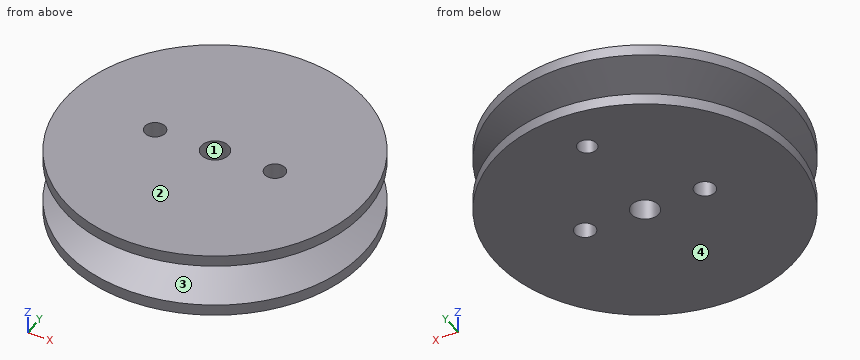
Autodesk Inventor part; units mm, degrees
ref_plane "Belt Plane" through (0, 32.131, 9.525) normal (0, 0, 1) x (1, 0, 0)
ref_plane "YZ Plane" through (0, 0, 0) normal (1, 0, 0) x (0, 1, 0)
ref_plane "XZ Plane" through (0, 0, 0) normal (0, 1, 0) x (-1, 0, 0)
sketch "Main Sketch" plane through (0, 0, 0) normal (1, 0, 0) x (0, 1, 0)
  line L0 (0, 19.05) -> (43.815, 19.05)
  line L1 (43.815, 19.05) -> (43.815, 15.8043)
  line L2 (43.815, 15.8043) -> (32.131, 12.2321)
  line L3 (32.131, 12.2321) -> (32.131, 6.8179)
  line L4 (32.131, 6.8179) -> (43.815, 3.2457)
  line L5 (43.815, 3.2457) -> (43.815, 0)
  line L6 (43.815, 0) -> (0, 0)
  line L7 (40.64, 14.8336) -> (40.64, 4.2164) construction
  line L8 (32.131, 9.525) -> (40.64, 9.525) construction
  line L9 (43.815, 15.8043) -> (43.815, 3.2457)
  line L10 (0, -4) -> (0, 24)
  line L11 (0, 0) -> (0, 19.05)
  dimension "d0" = 10.6172
  dimension "d1" = 34
  dimension "d2" = 3.175
  dimension "d6" = 19.05
  dimension "d21" = 81.28
  dimension "d25" = 11.684
  dimension "d27" = 9.525
ref_plane "Belt Plane" through (0, 32.131, 9.525) normal (0, 0, 1) x (1, 0, 0)
revolve "Body" add sketch "Main Sketch" angle 360 about axis through (0, 0, -10) along (0, 0, 1)
revolve "Groove" cut sketch "Main Sketch" angle 360 about axis through (0, 0, -10) along (0, 0, 1) contours L9 L4 L3 L2
fillet "Fillet External" [suppressed]
fillet "Fillet Internal" [suppressed]
pattern_of_one "Groove Pattern"
sketch "Sketch2" plane through (0, 0, 0) normal (0, 0, -1) x (-1, 0, 0)
  circle A0 centre (0, 0) radius 43.815
  line L0 (0, 0) -> (0, 30) construction
  circle A1 centre (0, 30) radius 2.75
  dimension "d28" = 5.5
  dimension "d29" = 30
extrude "Extrusion1" cut sketch "Sketch2" against normal blind 5 contours A1
sketch "Sketch3" plane through (0, 0, 19.05) normal (0, 0, 1) x (1, 0, 0)
  circle A0 centre (0, 0) radius 43.815
  circle A1 centre (0, 0) radius 4
  line L0 (-17.5, 0) -> (17.5, 0) construction
  circle A2 centre (-17.5, 0) radius 3
  circle A3 centre (17.5, 0) radius 3
  dimension "d32" = 8
  dimension "d33" = 35
  dimension "d34" = 6
extrude "Extrusion2" cut sketch "Sketch3" against normal through all contours A1 | A2 | A3
equation "\"d0\" = da_Bw"
equation "\"d1\" = da_Alfa"
equation "\"d2\" = da_c"
equation "\"d21\" = da_Dw"
equation "\"d25\" = da_Hd"
equation "\"d27\" = da_Se"
equation "\"da_r1\" = 0"
equation "\"da_r2\" = 0"
equation "\"d18\" = da_Sg"
equation "\"d5\" = da_Se"
equation "\"da_Bw\" = 10.6172"
equation "\"da_Alfa\" = 34deg"
equation "\"da_c\" = 3.175"
equation "\"da_Dw\" = 81.28"
equation "\"da_Hd\" = 11.684"
equation "\"da_Se\" = 9.525"
equation "\"da_Sg\" = 15.875"
properties part number "Grooved Pulley1" material "Steel"
Input: part model. Units: mm. Frame: model coordinates. Face numbers are marked on the shaded views. Coordinates: 2 decimals unless noted, no trailing zeros. Write each loop counter-clockwise with the first axis right and the second up, starting at its lowest first coordinate (ties: lowest second). Pieces come first, ordered by that corner, then holes.
1) Pin query (flat end, axial travel): pin 1 Ø2 at (y, z) = (5, 16) entering from -X; pin 2 Ø8 at (y, z) = (-15.5, 15.5) entering from -X; pin 3 Ø3.5 at (x, y) = (17.5, 0) entering from +Z; pin 4 Ø4 at (x, z) = (-22, 3.5) entering from -Y. Return the tip coordinate at first contact, or that it passes through.
2) Section D-D on z = 14.5. Output: boundary loops of the cut face in (x, y), and give its area (3 significant figures).
3) Section C-C on z = 9.5. Output: boundary loops of the cut face in (x, y).
4) Section B-B on y = 0. Output: boundary loops of the cut face in (x, z) (3 decimals).
5) Section A-A on x = 0. Output: boundary loops of the cut face in (y, z) (3 decimals).
6) Mould query, pull axis Z, two halves, no side actions, for the marked faces 1, 2, 3 and 4. Classes: pulls with the +Z half, pulls with the -Z half, needs draft (parallel to the pull), parting line crosses it, or undercut.
7) Material intervals for line 1 along Y through (x, z) = (0, 1.35) (3 decimals); line 2 along Y through (x, z) = (0, 11.5); line 3 along Z through (x, y) = (9, 36.5), sorted ascending.
Check result:
1. pin 1: stops at x = -43.63
1. pin 2: stops at x = -42.28
1. pin 3: passes through
1. pin 4: stops at y = -38.98
2. outline: circle Ø79.1 at (0, 0); hole circle Ø6 at (-17.5, 0); hole circle Ø8 at (0, 0); hole circle Ø6 at (17.5, 0)
2. area: 4,810 mm2
3. outline: circle Ø64.26 at (0, 0); hole circle Ø6 at (-17.5, 0); hole circle Ø8 at (0, 0); hole circle Ø6 at (17.5, 0)
4. outline: (-43.815, 0) - (-20.5, 0) - (-20.5, 19.05) - (-43.815, 19.05) - (-43.815, 15.804) - (-32.131, 12.232) - (-32.131, 6.818) - (-43.815, 3.246) - close; (-14.5, 0) - (-4, 0) - (-4, 19.05) - (-14.5, 19.05) - close; (4, 0) - (14.5, 0) - (14.5, 19.05) - (4, 19.05) - close; (20.5, 0) - (43.815, 0) - (43.815, 3.246) - (32.131, 6.818) - (32.131, 12.232) - (43.815, 15.804) - (43.815, 19.05) - (20.5, 19.05) - close
5. outline: (-43.815, 0) - (-4, 0) - (-4, 19.05) - (-43.815, 19.05) - (-43.815, 15.804) - (-32.131, 12.232) - (-32.131, 6.818) - (-43.815, 3.246) - close; (4, 0) - (27.25, 0) - (27.25, 5) - (32.75, 5) - (32.75, 0) - (43.815, 0) - (43.815, 3.246) - (32.131, 6.818) - (32.131, 12.232) - (43.815, 15.804) - (43.815, 19.05) - (4, 19.05) - close
6. face 1: needs draft
6. face 2: pulls with the +Z half
6. face 3: undercut
6. face 4: pulls with the -Z half
7. line 1: y = -43.815 to -4, 4 to 27.25, 32.75 to 43.815
7. line 2: y = -32.13 to -4, 4 to 32.13
7. line 3: z = 0 to 5.15, 13.9 to 19.05
